Part print with two shaded views. Sizes in mm from the minimum x, y, z corner. Round coordinates to 2 decimals unless told otherwise and drop trailing zeros. Write each loop counter-clockwise with the first axis right and the second up, starting at its lowest first coordinate (ties: lowest second). Pieces come first, ordered by that corner, then holes. Notation, with made-up numbers: (-12, -20) -> (-6, -20) arc R30 ccw to (-6, 16) -> close; hole circle Ø9 at (67, -26.5). An arc over 180 degrees is marked (long way). Return JSON: item names as keys, results as strings. Group by question number.
(1) Drill centre lines: L1, parallel to Z at x = 27, y = 1.1 (1 decimal); L2, parallel to Z at x = 29, y = 2.15 (1 decimal); L3, parallel to Z at x = 8, y = 1.55. Where is each one in solid material? Low to high. Write a range as from..to.
(2) Saw through at B-B (x = 3.5). List the corners of the cut face in (y, z).
(3) Saw through at D-D (x = 28.5). List the corners of the cut face in (y, z).
(4) Mould opens along Z. For the marked faces 1, 2 and 3 say: +Z half, -Z half, draft (parallel to the pull), parting line (faces both ways), or undercut.
(5) Saw through at C-C (y = 2.1). List the corners of the cut face in (x, z), plus the area to 3 significant figures.
(6) Saw through at A-A (z = 15). List the corners of the cut face in (x, y).
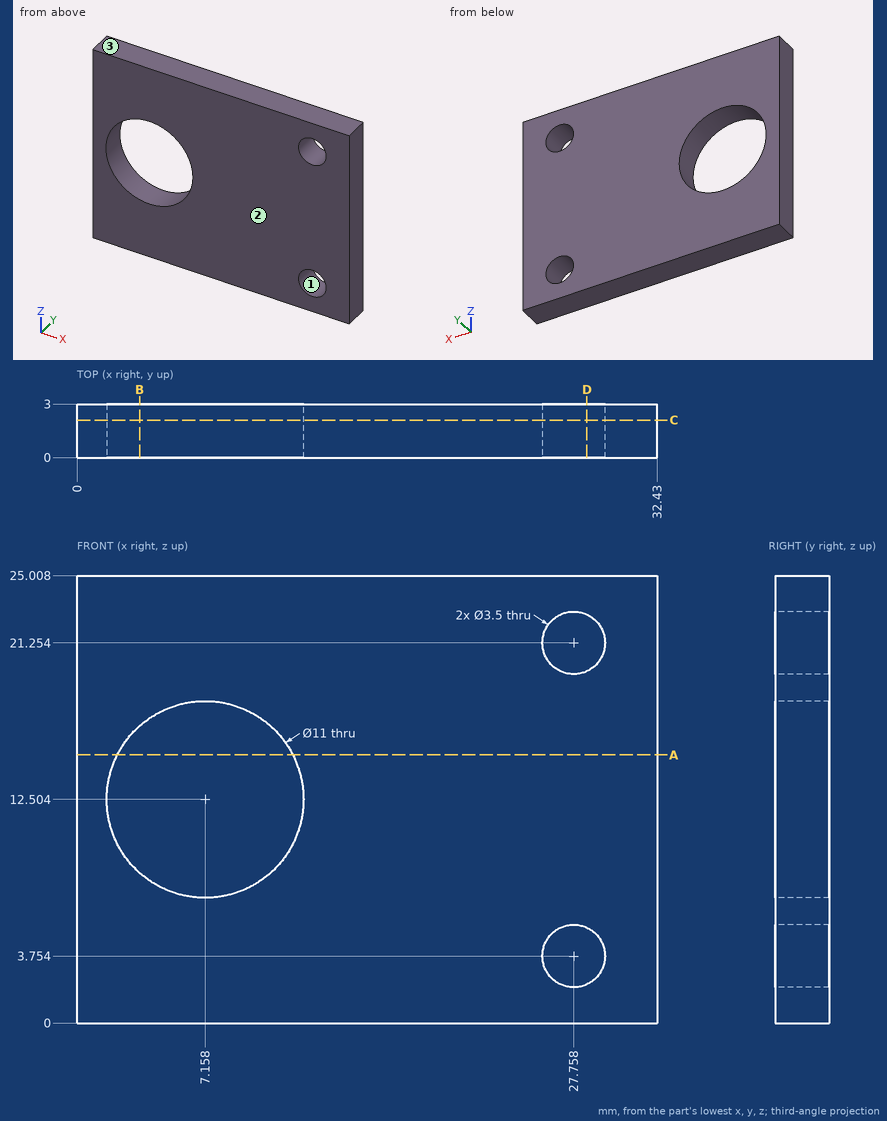
Computed values:
{
 "1": {"L1": "0..2.2, 5.3..19.7, 22.8..25", "L2": "0..2.5, 5..20, 22.5..25", "L3": "0..7.07, 17.94..25.01"},
 "2": {"outline": "(0, 0) -> (3, 0) -> (3, 8.4) -> (0, 8.4) -> close; (0, 16.61) -> (3, 16.61) -> (3, 25.01) -> (0, 25.01) -> close"},
 "3": {"outline": "(0, 0) -> (3, 0) -> (3, 2.17) -> (0, 2.17) -> close; (0, 5.34) -> (3, 5.34) -> (3, 19.67) -> (0, 19.67) -> close; (0, 22.84) -> (3, 22.84) -> (3, 25.01) -> (0, 25.01) -> close"},
 "4": {"face 1": "undercut", "face 2": "draft", "face 3": "+Z half"},
 "5": {"outline": "(0, 0) -> (32.43, 0) -> (32.43, 25.01) -> (0, 25.01) -> close; hole circle Ø11 at (7.16, 12.5); hole circle Ø3.5 at (27.76, 3.75); hole circle Ø3.5 at (27.76, 21.25)", "area": "697 mm2"},
 "6": {"outline": "(0, 0) -> (2.26, 0) -> (2.26, 3) -> (0, 3) -> close; (12.06, 0) -> (32.43, 0) -> (32.43, 3) -> (12.06, 3) -> close"}
}
